Build history of the part. All positions in model axes, mm. A direction names the side the tool comes from. Round coordinates to 2 decimals unless told otherwise and drop trailing zeros. Write each loop counter-clockwise with the first axis right and the second up, starting at its lowest first coordinate (ties: lowest second). Pieces come first, ordered by that corner, then holes.
from build123d import *

# Parameters (mm, degrees)
SKETCH_R    = 35
SKETCH_R_2  = 1.5625
PAD_DEPTH   = 12
FILLET_R    = 3
FILLET001_R = 3


with BuildPart() as part:
    # Sketch → Pad (new body)
    with BuildSketch(Plane.XY):
        Polygon((0, 0), (200, 0), (200, 200), (160, 200), (160, 130), (40, 130), (40, 200), (0, 200), align=None)
        with Locations((100, 65)):
            Circle(SKETCH_R, mode=Mode.SUBTRACT)
        with Locations((45, 115)):
            Circle(SKETCH_R_2, mode=Mode.SUBTRACT)
        with Locations((45, 15)):
            Circle(SKETCH_R_2, mode=Mode.SUBTRACT)
        with Locations((155, 115)):
            Circle(SKETCH_R_2, mode=Mode.SUBTRACT)
        with Locations((155, 15)):
            Circle(SKETCH_R_2, mode=Mode.SUBTRACT)
        with Locations((185, 30)):
            Circle(SKETCH_R_2, mode=Mode.SUBTRACT)
        with Locations((135.355339, 100.355339)):
            Circle(SKETCH_R_2, mode=Mode.SUBTRACT)
        with Locations((64.644661, 29.644661)):
            Circle(SKETCH_R_2, mode=Mode.SUBTRACT)
        with Locations((64.644661, 100.355339)):
            Circle(SKETCH_R_2, mode=Mode.SUBTRACT)
        with Locations((135.355339, 29.644661)):
            Circle(SKETCH_R_2, mode=Mode.SUBTRACT)
        with Locations((175, 20)):
            Circle(SKETCH_R_2, mode=Mode.SUBTRACT)
        with Locations((175, 40)):
            Circle(SKETCH_R_2, mode=Mode.SUBTRACT)
        with Locations((185, 50)):
            Circle(SKETCH_R_2, mode=Mode.SUBTRACT)
        with Locations((175, 90)):
            Circle(SKETCH_R_2, mode=Mode.SUBTRACT)
        with Locations((175, 110)):
            Circle(SKETCH_R_2, mode=Mode.SUBTRACT)
        with Locations((185, 80)):
            Circle(SKETCH_R_2, mode=Mode.SUBTRACT)
        with Locations((185, 100)):
            Circle(SKETCH_R_2, mode=Mode.SUBTRACT)
        with Locations((15, 30)):
            Circle(SKETCH_R_2, mode=Mode.SUBTRACT)
        with Locations((25, 20)):
            Circle(SKETCH_R_2, mode=Mode.SUBTRACT)
        with Locations((25, 40)):
            Circle(SKETCH_R_2, mode=Mode.SUBTRACT)
        with Locations((15, 50)):
            Circle(SKETCH_R_2, mode=Mode.SUBTRACT)
        with Locations((25, 90)):
            Circle(SKETCH_R_2, mode=Mode.SUBTRACT)
        with Locations((25, 110)):
            Circle(SKETCH_R_2, mode=Mode.SUBTRACT)
        with Locations((15, 80)):
            Circle(SKETCH_R_2, mode=Mode.SUBTRACT)
        with Locations((15, 100)):
            Circle(SKETCH_R_2, mode=Mode.SUBTRACT)
        with Locations((25, 180)):
            Circle(SKETCH_R_2, mode=Mode.SUBTRACT)
        with Locations((25, 160)):
            Circle(SKETCH_R_2, mode=Mode.SUBTRACT)
        with Locations((15, 170)):
            Circle(SKETCH_R_2, mode=Mode.SUBTRACT)
        with Locations((175, 180)):
            Circle(SKETCH_R_2, mode=Mode.SUBTRACT)
        with Locations((175, 160)):
            Circle(SKETCH_R_2, mode=Mode.SUBTRACT)
        with Locations((185, 170)):
            Circle(SKETCH_R_2, mode=Mode.SUBTRACT)
        with Locations((15, 120)):
            Circle(SKETCH_R_2, mode=Mode.SUBTRACT)
        with Locations((15, 150)):
            Circle(SKETCH_R_2, mode=Mode.SUBTRACT)
        with Locations((185, 120)):
            Circle(SKETCH_R_2, mode=Mode.SUBTRACT)
        with Locations((185, 150)):
            Circle(SKETCH_R_2, mode=Mode.SUBTRACT)
    extrude(amount=PAD_DEPTH)

    # Fillet
    fillet_edges = [part.edges().sort_by_distance(p)[0] for p in [
        (0, 0, 6),
        (200, 0, 6),
        (0, 200, 6),
        (160, 200, 6),
        (40, 200, 6),
        (200, 200, 6),
    ]]
    fillet(fillet_edges, radius=FILLET_R)

    # Fillet001
    fillet001_edges = [part.edges().sort_by_distance(p)[0] for p in [
        (160, 130, 6),
        (40, 130, 6),
    ]]
    fillet(fillet001_edges, radius=FILLET001_R)


solid = part.part
1) Slice it at B-B (x = 100). Write the cut outline in (y, z).
Results:
outline: (0, 0) - (30, 0) - (30, 12) - (0, 12) - close; (100, 0) - (130, 0) - (130, 12) - (100, 12) - close
2) Slice it at A-A (y = 186.5). Write the cut outline in (x, z), plus the area to 3 significant figures.
Results:
outline: (0, 0) - (40, 0) - (40, 12) - (0, 12) - close; (160, 0) - (200, 0) - (200, 12) - (160, 12) - close
area: 960 mm2
3) Slice it at C-C (x = 149). Write the cut outline in (y, z).
Results:
outline: (0, 0) - (130, 0) - (130, 12) - (0, 12) - close
4) Pin check, flat tips, straight feed: pin 1 Ø1.9 at (x, y) = (25, 20) entering from +Z; pin 2 Ø3 at (x, z) = (109.5, 2.5) entering from +Y. Stop position of each tip, or through.
Results:
pin 1: passes through
pin 2: stops at y = 130
5) Mould opens along Y. For faces 3 (the flat face through (101, 130, 6)), 4 (the flat face through (200, 99, 6)), 5 (the cylindrical face through (118.82, 94.51, 5.92)) say: released by +Y, released by -Y, zero draft, split by the parting line, or undercut.
Results:
face 3: released by +Y
face 4: zero draft
face 5: undercut
6) Which spindle directions (+Z, -Z, +X, -X, +Y, -Y) get a long thin tool onto all of the face, cutting with end or side? Do faces 1 (the flat face through (99, 101, 12)), 2 (the flat face through (40, 165, 6)). Say none if no direction does.
Results:
face 1: +Z, +X, -X, +Y, -Y
face 2: +Z, -Z, +Y
7) Slice it at D-D (z = 6.5). Count the separate pieces of the cut face and the enclosed holes in it, plus the area to 3 significant figures.
Results:
separate pieces: 1
enclosed holes: 35
area: 27,500 mm2
8) Wall check: L1, parallel to X at y = 110, z = 4; L2, parallel to X at y = 14, z = 7.25; L3, parallel to X at y = 157.5, z = 1. Give the ranges that are in metal, low to high.
Results:
L1: x = 0 to 23.44, 26.56 to 173.44, 176.56 to 200
L2: x = 0 to 43.8, 46.2 to 153.8, 156.2 to 200
L3: x = 0 to 40, 160 to 200
